from build123d import *

# Parameters (mm, degrees)
SKETCH1_W               = 25
SKETCH1_H               = 46
BOSS_EXTRUDE1_DEPTH     = 18
SKETCH2_W               = 7
SKETCH2_H               = 3
BOSS_EXTRUDE2_DEPTH     = 10
CUT_EXTRUDE1_DEPTH      = 10
CUT_EXTRUDE2_DEPTH      = 4
CUT_EXTRUDE2_DEPTH_BACK = 4
SKETCH5_R               = 12.5
CUT_EXTRUDE3_DEPTH      = 7
CUT_EXTRUDE3_DEPTH_BACK = 7
CUT_EXTRUDE4_REACH      = 61.372
SKETCH8_R               = 1.75
SKETCH9_W               = 6.4
SKETCH9_H               = 38
CUT_EXTRUDE5_DEPTH      = 36
SKETCH10_W              = 7.5
SKETCH10_H              = 10
SKETCH10_W_2            = 2.5
SKETCH10_W_3            = 5.5
CUT_EXTRUDE6_DEPTH      = 32
FILLET1_R               = 4
FILLET2_R               = 2
CUT_EXTRUDE7_DEPTH      = 32


with BuildPart() as part:
    # Sketch1 → Boss-Extrude1 (new body)
    with BuildSketch(Plane.XY):
        with Locations((-12.5, 23)):
            Rectangle(SKETCH1_W, SKETCH1_H)
    extrude(amount=BOSS_EXTRUDE1_DEPTH)

    # Sketch2 → Boss-Extrude2 (add)
    with BuildSketch(Plane.XY.offset(18)):
        with Locations((-11, 44.5)):
            Rectangle(SKETCH2_W, SKETCH2_H)
    extrude(amount=BOSS_EXTRUDE2_DEPTH)

    # Sketch3 → Cut-Extrude1 (cut)
    with BuildSketch(Plane(origin=(0, 46, 0), x_dir=(1, 0, 0), z_dir=(0, 1, 0))):
        with BuildLine():
            Line((-12.75, -28), (-12.75, -20))
            ThreePointArc((-12.75, -20), (-11, -18.25), (-9.25, -20))
            Line((-9.25, -20), (-9.25, -28))
            ThreePointArc((-9.25, -28), (-11, -29.75), (-12.75, -28))
        make_face()
    extrude(amount=-CUT_EXTRUDE1_DEPTH, mode=Mode.SUBTRACT)

    # Sketch5 → Cut-Extrude2 (cut, two sides: drawn at the far end of the back side and taken through both)
    with BuildSketch(Plane.ZY.offset(11).offset(-CUT_EXTRUDE2_DEPTH_BACK)):
        with Locations((10.5, 22)):
            Circle(SKETCH5_R)
    extrude(amount=CUT_EXTRUDE2_DEPTH + CUT_EXTRUDE2_DEPTH_BACK, mode=Mode.SUBTRACT)

    # Sketch7 → Cut-Extrude3 (cut, two sides: drawn at the far end of the back side and taken through both)
    with BuildSketch(Plane.ZY.offset(11).offset(-CUT_EXTRUDE3_DEPTH_BACK)):
        with BuildLine():
            Line((10.5, 26), (19.804509891, 26))
            ThreePointArc((19.804509891, 26), (23.804509891, 22), (19.804509891, 18))
            Line((19.804509891, 18), (10.5, 18))
            ThreePointArc((10.5, 18), (6.5, 22), (10.5, 26))
        make_face()
    extrude(amount=CUT_EXTRUDE3_DEPTH + CUT_EXTRUDE3_DEPTH_BACK, mode=Mode.SUBTRACT)

    # Sketch8 → Cut-Extrude4 (cut, up to next)
    with BuildSketch(Plane.ZY.offset(25), mode=Mode.PRIVATE) as cut_extrude4_sk1:
        with Locations((5.8, 5)):
            Circle(SKETCH8_R)
    cut_extrude4_tool1 = extrude(cut_extrude4_sk1.sketch, amount=-CUT_EXTRUDE4_REACH, mode=Mode.PRIVATE) & part.part
    add(cut_extrude4_tool1.solids().sort_by_distance((-25, 5, 5.8))[0], mode=Mode.SUBTRACT)

    # Sketch9 → Cut-Extrude5 (cut)
    with BuildSketch(Plane.ZY.offset(25)):
        with Locations((14.8, 19)):
            Rectangle(SKETCH9_W, SKETCH9_H)
    extrude(amount=-CUT_EXTRUDE5_DEPTH, mode=Mode.SUBTRACT)

    # Sketch10 → Cut-Extrude6 (cut)
    with BuildSketch(Plane.XY.offset(11.6)):
        with Locations((-11, 5)):
            Rectangle(SKETCH10_W, SKETCH10_H)
        with Locations((-1.25, 5)):
            Rectangle(SKETCH10_W_2, SKETCH10_H)
        with Locations((-22.25, 5)):
            Rectangle(SKETCH10_W_3, SKETCH10_H)
    extrude(amount=-CUT_EXTRUDE6_DEPTH, mode=Mode.SUBTRACT)

    # Fillet1
    fillet1_edges = [part.edges().sort_by_distance(p)[0] for p in [
        (-17.125, 0, 11.6),
        (-4.875, 0, 0),
        (-4.875, 0, 11.6),
        (-17.125, 0, 0),
    ]]
    fillet(fillet1_edges, radius=FILLET1_R)

    # Fillet2
    fillet2_edges = [part.edges().sort_by_distance(p)[0] for p in [
        (-11, 10, 0),
        (-1.25, 10, 0),
        (-1.25, 10, 11.6),
        (-22.25, 10, 0),
        (-22.25, 10, 11.6),
        (-12.5, 46, 0),
    ]]
    fillet(fillet2_edges, radius=FILLET2_R)

    # Sketch11 → Cut-Extrude7 (cut)
    with BuildSketch(Plane.XY.offset(18)):
        with BuildLine():
            Line((-19.5, 41), (-19.5, 46.514894744))
            Line((-19.5, 46.514894744), (-16, 46.514894744))
            Line((-16, 46.514894744), (-16, 41))
            ThreePointArc((-16, 41), (-17.75, 39.25), (-19.5, 41))
        make_face()
        with BuildLine():
            Line((-6, 41), (-6, 46.514894744))
            Line((-6, 46.514894744), (-2.5, 46.514894744))
            Line((-2.5, 46.514894744), (-2.5, 41))
            ThreePointArc((-2.5, 41), (-4.25, 39.25), (-6, 41))
        make_face()
    extrude(amount=-CUT_EXTRUDE7_DEPTH, mode=Mode.SUBTRACT)


solid = part.part
Can you work these out from the model? Positions are in its coordinate system, mm. A direction names the side the tool comes from. Give positions to 0.01 mm unless a question says otherwise; leave off trailing zeros. Order: outer loops, then holes, each group sorted by start corner. A loop starts at its lowest first (then second) coordinate and runs counter-clockwise, first axis right, second up. Notation, with made-up numbers: M 50.5,1.5 L 88.5,1.5 A33 ccw 88.5,33.5 Z; hole C 6.5,36 d1. An arc over 180 degrees is marked long. Use one line per item in the form item = value. Start each with the question number.
Item 1: Will these pins go through, and if not, where does the flat tip stop? pin 1 Ø4.5 at (y, z) = (5, 5.8) entering from -X; pin 2 Ø6 at (x, z) = (-23, 5.5) entering from -Y; pin 3 Ø10 at (x, y) = (-8.5, 7.5) entering from +Z; pin 4 Ø1 at (x, y) = (-14, 5) entering from -Z.
Item 2: If we section it at D-D (y = 4.5): Write out the boundary of the cut face in (x, z), then the cut area to 3 significant figures.
Item 3: If we section it at A-A (z = 4.75): State how many separate pieces and enclosed holes the cut face has, then the cut area to 3 significant figures.
Item 4: We'd pull the mould along Y, two halves only. Please class faces 1 (the cylindrical face through (-10.944, 33.272, 5.097)), 2 (the cylindrical face through (-1.23, 10.6, 0.57)), 3 (the flat face through (-18.2, 20.8, 11.6)): +Y half, -Y half, draft (parallel to the pull), parting line (faces both ways), or undercut.
Item 5: If we section it at B-B (y = 22): Write out the boundary of the cut face in (x, z), then the cut area to 3 significant figures.
Item 6: If I drill on line 1 along X through (y, z) = (41, 3.5); line 2 along X through (y, z) = (18, 4); line 3 along X through (y, z) = (23, 8), over which ranges is the centre line in solid material (lowest first)?
Item 7: If we section it at C-C (x = -19): Write out the boundary of the cut face in (y, z).
Item 8: For faces 4 (the flat face through (-13, 38, 15)), 5 (the flat face through (-16, 44, 9)), 6 (the flat face through (-7, 22, 6)), 7 (the flat face through (-11, 10, 5)), 8 (the flat face through (-12.75, 45, 24)), which set-ups out of +Z, -Z, +X, -X, +Y, -Y let a thin tool reach every point of the face, with its end or its side?
Outcome:
q1.pin_1 = -19.5
q1.pin_2 = 10
q1.pin_3 = 11.6
q1.pin_4 = through
q2.outline = M -19.5,0 L -14.75,0 L -14.75,4.12 L -19.5,4.12 Z; M -19.5,7.48 L -14.75,7.48 L -14.75,11.6 L -19.5,11.6 Z; M -7.25,0 L -2.5,0 L -2.5,4.12 L -7.25,4.12 Z; M -7.25,7.48 L -2.5,7.48 L -2.5,11.6 L -7.25,11.6 Z
q2.area = 78.3 mm2
q3.separate_pieces = 3
q3.enclosed_holes = 1
q3.area = 746 mm2
q4.face_1 = undercut
q4.face_2 = -Y half
q4.face_3 = draft
q5.outline = M -25,0 L -15,0 L -15,6.5 L -18,6.5 L -18,11.6 L -25,11.6 Z; M -7,0 L 0,0 L 0,11.6 L -4,11.6 L -4,6.5 L -7,6.5 Z
q5.area = 167 mm2
q6.line_1 = -25 to -19.5, -16 to -6, -2.5 to 0
q6.line_2 = -25 to -15, -7 to 0
q6.line_3 = -25 to -18, -4 to 0
q7.outline = M 0,4 A4 ccw 4,0 L 39.78,0 L 39.78,18 L 38,18 L 38,11.6 L 4,11.6 A4 ccw 0,7.6 Z; hole C 5,5.8 d3.5
q8.face_4 = +Z, +X, -X, -Y
q8.face_5 = +Z, -Z, +Y
q8.face_6 = +Z
q8.face_7 = +Z, -Z, -Y
q8.face_8 = +Z, +Y, -Y
